Read the model definition and answer for the solid it produces. Units are mm, in the model's axes. Face numbers are marked on the shaded views. A direction names the side the tool comes from. Coordinates: 2 decimals unless noted, no trailing zeros. Loops run counter-clockwise (first coordinate to the right, second up) from the corner with the lowest first, then second, coordinate; pieces in that order, holes last. Notation, with made-up numbers: M -12,49 L 0,49 A22 cw 0,70 Z; hole C 49,-24.75 d1. An arc over 180 degrees is marked long. Put each result on its own line as item: value.
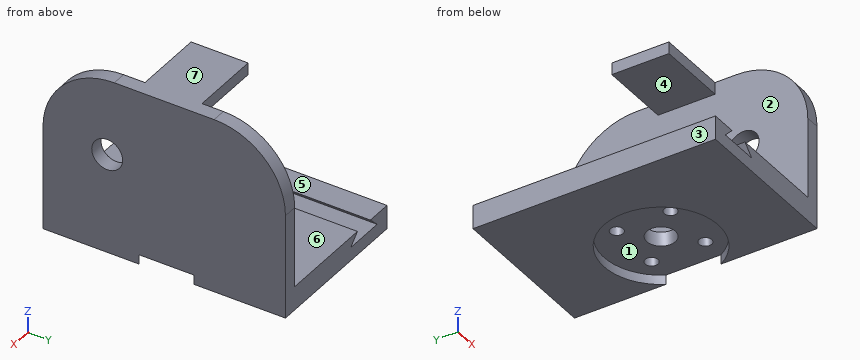
Solid Edge part; units mm, degrees
sketch "Sketch1" plane through (0, 0, 0) normal (0, 0, -1) x (-1, 0, 0)
  line L0 (5, 86.5) -> (5, 35.5)
  line L1 (-28, 35.5) -> (5, 35.5)
  line L2 (-28, 86.5) -> (-28, 35.5)
  line L3 (5, 86.5) -> (-28, 86.5)
  dimension "D1" = 5
  dimension "D2" = 28
extrude "Protrusion1" add sketch "Sketch1" along normal blind 5
sketch "Sketch2" plane through (8, 36.5, -5) normal (0, 0, -1) x (1, 0, 0)
  circle A0 centre (9.5, -25) radius 12
  dimension "D1" = 9.5
extrude "VaciadoExtruido_1" cut sketch "Sketch2" against normal blind 2
sketch "Sketch3" plane through (8, 86.5, -2) normal (0, 1, 0) x (1, 0, 0)
  line L0 (-7.6, -2) -> (-9.8, 0.2)
  line L1 (-9.8, 0.2) -> (-5.5, 0.2)
  line L2 (-1.2, 0.2) -> (-5.5, 0.2)
  line L3 (-3.4, -2) -> (-1.2, 0.2)
  line L4 (-3.4, -2) -> (-5.5, -2)
  line L5 (-7.6, -2) -> (-5.5, -2)
extrude "Cutout1" cut sketch "Sketch3" against normal through all
sketch "Sketch4" plane through (8, 86.5, -2.5) normal (0, 1, 0) x (1, 0, 0)
  line L0 (20, -34.5) -> (20, -2.5)
  line L1 (20, -2.5) -> (17, -2.5)
  line L2 (17, -2.5) -> (17, -34.5)
  line L3 (17, -34.5) -> (20, -34.5)
extrude "ProtrusiónExtruida_4" add sketch "Sketch4" against normal blind 51
hole "Agujero_10" at (17.5, 61.5, -3) direction (0, 0, 1) diameter 6 end up to next
sketch "Sketch5" plane through (16.75, 61.5, -3) normal (0, 0, -1) x (0, -1, 0)
  circle A0 centre (-5.6569, 4.9069) radius 1.35
  circle A1 centre (-5.6569, -6.4069) radius 1.35
  circle A2 centre (5.6569, 4.9069) radius 1.35
  circle A3 centre (5.6569, -6.4069) radius 1.35
extrude "Cutout2" cut sketch "Sketch5" against normal through all
fillet "Redondeo_1" radius 15 1 edges at (26.5, 86.5, 32)
fillet "Redondeo_2" radius 15 1 edges at (26.5, 35.5, 32)
sketch "Sketch6" plane through (28, 61, 13.5) normal (1, 0, 0) x (0, -1, 0)
  circle A0 centre (12, -2.5) radius 3.25
extrude "Cutout3" cut sketch "Sketch6" against normal through all
sketch "Sketch7" plane through (25, 61, 16) normal (-1, 0, 0) x (0, 1, 0)
  line L0 (6, -13.5) -> (-6, -13.5)
  line L1 (-6, -13.5) -> (-6, -16)
  line L2 (-6, -16) -> (6, -16)
  line L3 (6, -16) -> (6, -13.5)
extrude "ProtrusiónExtruida_5" add sketch "Sketch7" along normal blind 15
properties material "Aluminio, 7075-T6"
1) Given pin 1 Ø2.5 at (x, y) = (23.16, 55.84) entering from -Z; pin 2 Ø5 at (x, y) = (17, 46.5) entering from +Z; pin 3 Ø3.5 at (x, y) = (11.84, 55.84) entering from -Z; pin 4 Ø1 at (y, z) = (47, 17.5) entering from +X, each flat-ended and moving along its own axis, determine where each tip first touches the part or whether it passes through.
Answer list:
pin 1: stops at z = 29.5
pin 2: stops at z = 0
pin 3: stops at z = -3
pin 4: passes through
2) Find section B-B, the plane y = 61.5. Write down the section's boundary in (x, z), plus the area to 3 significant figures.
Answer list:
outline: M -5,-5 L 5.5,-5 L 5.5,-3 L 14.5,-3 L 14.5,0 L 4.6,0 L 6.8,-2.2 L -1.8,-2.2 L 0.4,0 L -5,0 Z; M 10,29.5 L 25,29.5 L 25,0 L 20.5,0 L 20.5,-3 L 28,-3 L 28,32 L 10,32 Z
area: 221 mm^2
3) Find section C-C, the plane z = -1. Write down the section's boundary in (x, y), plus the area to 3 significant figures.
Answer list:
outline: M -5,35.5 L -0.6,35.5 L -0.6,86.5 L -5,86.5 Z; M 5.6,35.5 L 28,35.5 L 28,86.5 L 5.6,86.5 Z; hole C 11.84,55.84 d2.7; hole C 11.84,67.16 d2.7; hole C 17.5,61.5 d6; hole C 23.16,55.84 d2.7; hole C 23.16,67.16 d2.7
area: 1,320 mm^2
4) Which of the six approach directions +Z, -Z, +X, -X, +Y, -Y give full straight-line access (tool end or side, diameter ignored) to the marked faces 5, 6 and 7?
Answer list:
face 5: +Z, -X, +Y, -Y
face 6: -X, +Y, -Y
face 7: +Z, +X, -X, +Y, -Y
5) Find section A-A, the plane x = 17.5. Write down the section's boundary in (y, z), plus the area to 3 significant figures.
Answer list:
outline: M 35.5,-5 L 49.5,-5 L 49.5,-3 L 58.5,-3 L 58.5,0 L 35.5,0 Z; M 55,29.5 L 67,29.5 L 67,32 L 55,32 Z; M 64.5,-3 L 73.5,-3 L 73.5,-5 L 86.5,-5 L 86.5,0 L 64.5,0 Z
area: 219 mm^2
6) Determine the mould class of the marked faces 1, 2, 3 and 4 for opening direction Z: released by +Z, released by -Z, zero draft, split by the parting line, or undercut.
Answer list:
face 1: released by -Z
face 2: undercut
face 3: zero draft
face 4: undercut
7) Straight lines are drawn through the part: line 1 (Y direction, x = 27, z = 16); line 2 (Z direction, x = 21, y = 62); line 3 (Z direction, x = 1, y = 81). For each, find the intervals that lie inside material, in ascending order. Write a range as [from, to].
Answer list:
line 1: y = [35.5, 45.75], [52.25, 86.5]
line 2: z = [-3, 0], [29.5, 32]
line 3: z = [-5, -2.2]
8) Find section D-D, the plane y = 53.5. Write down the section's boundary in (x, z), plus the area to 3 significant figures.
Answer list:
outline: M -5,-5 L 8.56,-5 L 8.56,-3 L 26.44,-3 L 26.44,-5 L 28,-5 L 28,32 L 25,32 L 25,0 L 4.6,0 L 6.8,-2.2 L -1.8,-2.2 L 0.4,0 L -5,0 Z
area: 211 mm^2
